Study the drawing (mm; zero at the part's minimum x, y, z) and answer. A direction names the side the tool comes from. Give positions to 0.01 mm unless a question says otherwise; leave off trailing zeros. Loops run counter-clockwise (first coordinate to the right, second up) from the corner with the lowest first, then second, coordinate; pieces in that order, holes last. Notation, with made-up numbers: (5.25, 66) - (55.25, 66) arc R23 ccw to (55.25, 86) - close; hole circle Ø10 at (-2, 78). An arc over 180 degrees is marked (long way). Write item = value, one per line. Start each with the question number.
1) Which of the six approach directions +Z, -Z, +X, -X, +Y, -Y give full straight-line access (tool end or side, diameter ignored) to the marked faces 1, 2 and 3?
2) Flat-ended cylindrical pins translate along their axes: P1, Ø0.5, axis at x = 0.5, y = 2.5, coming from the +Z side; P2, Ø2, axis at x = 7.5, z = 3, coming from the +Y side; P3, Ø1.1, axis at x = 0.5, y = 1, coming from the -Z side; P4, Ø1.1, axis at x = 0.5, z = 2, coming from the +Y side. Find the tip coordinate at first contact, or state that the pin passes through.
3) Consider probe 1 along X at (y, z) = (2.85, 1.8); probe 2 along X at (y, z) = (4.05, 4); probe 3 along Z at (x, y) = (15, 2.75). Determine where each line is inside the solid, lowest interval first.
4) The part is cut by section C-C on x = 8.25. Write down the section's boundary in (y, z).
5) The part is cut by section A-A on y = 2.75. Write down the section's boundary in (x, z).
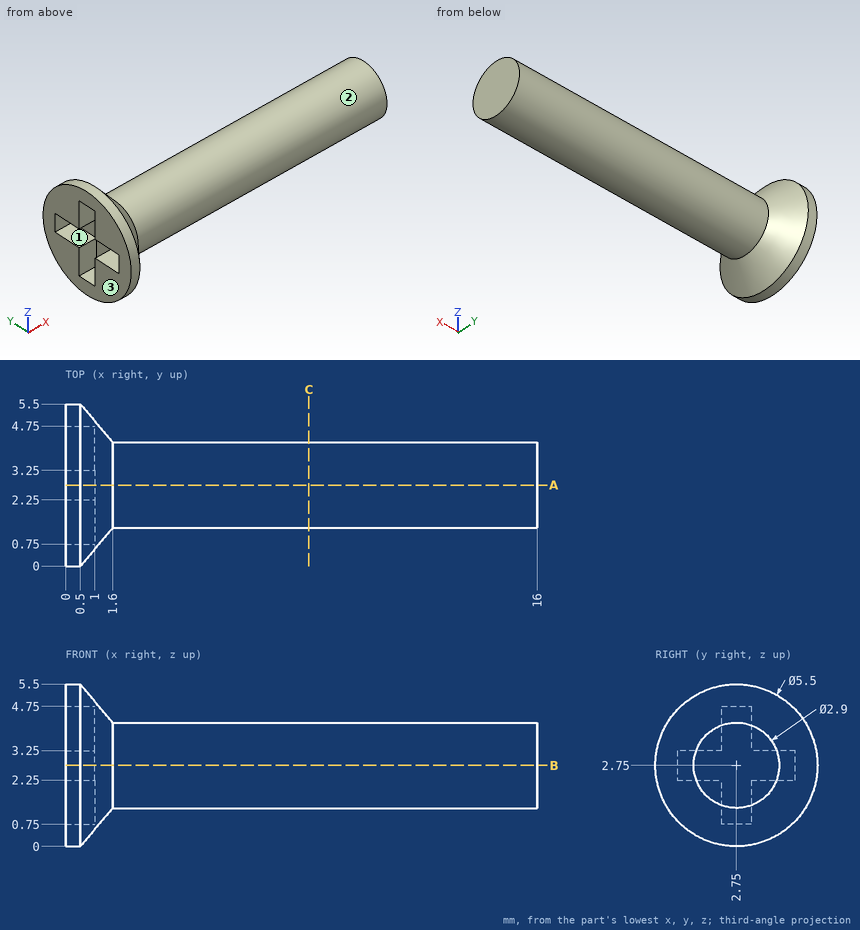
Answer below:
q1.face_1 = -X
q1.face_2 = +X
q1.face_3 = +Z, -Z, -X, +Y, -Y
q2.P1 = 5.5
q2.P2 = 4.2
q2.P3 = 0.28
q2.P4 = 5.49
q3.probe_1 = 1 to 16
q3.probe_2 = 0 to 1.3
q3.probe_3 = 1.3 to 4.2
q4.outline = circle Ø2.9 at (2.75, 2.75)
q5.outline = (0, 0) - (0.5, 0) - (1.6, 1.3) - (16, 1.3) - (16, 4.2) - (1.6, 4.2) - (0.5, 5.5) - (0, 5.5) - (0, 4.75) - (1, 4.75) - (1, 0.75) - (0, 0.75) - close
